Check sheet for the drawn part. Datum: minimum x, y, z corner. Units: mm. A direction names the side the tool comes from. Coordinates: 2 decimals unless noted, no trailing zeros. Loops run counter-clockwise (first coordinate to the right, second up) from the corner with the lowest first, then second, coordinate; pieces in that order, holes last.
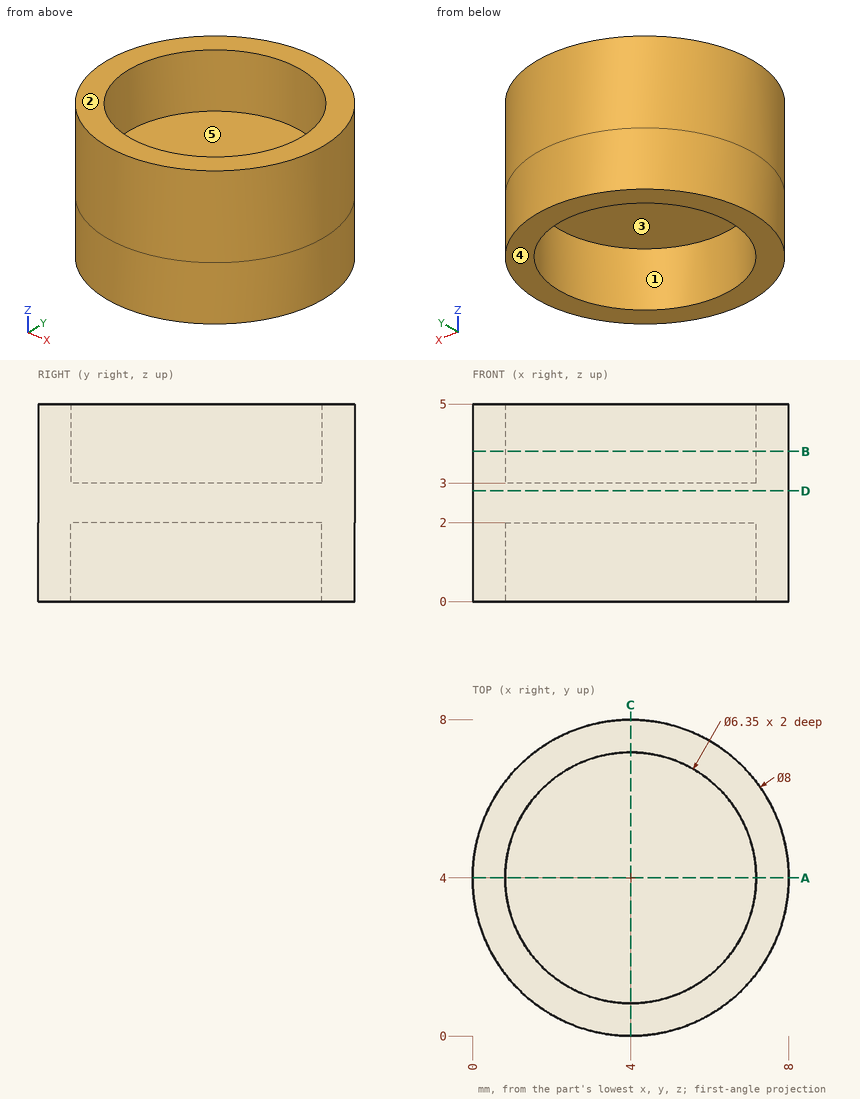
1) Section check A-A on y = 4. Enter the section's corners in (x, z) (3 decimals), plus the area to 3 significant figures.
Answer sheet:
outline: (0, 0) - (0.825, 0) - (0.825, 2) - (7.175, 2) - (7.175, 0) - (8, 0) - (8, 5) - (7.175, 5) - (7.175, 3) - (0.825, 3) - (0.825, 5) - (0, 5) - close
area: 14.6 mm2
2) Section check D-D on z = 2.8. Enter the section's corners in (x, y).
Answer sheet:
outline: circle Ø8 at (4, 4)
3) Depth check by flat-ended pin: pin 1 (1.9 mm diameter, centred on x = 5.5, y = 3, fed in from +Z); pin 2 (1 mm diameter, centred on x = 4.5, y = 5, fed in from -Z); pin 3 (2 mm diameter, centred on x = 7, z = 3, fed in from -Y). Enter the tip coordinate at first touch or a pass-through.
Answer sheet:
pin 1: stops at z = 3
pin 2: stops at z = 2
pin 3: stops at y = 0.54
4) Mould release check, pull along X, two halves, no side actions. Record for the marked faces 1, 2 and 3: +X half, -X half, draft (parallel to the pull), parting line (faces both ways), or undercut.
Answer sheet:
face 1: undercut
face 2: draft
face 3: undercut
5) Set-up check for the marked faces 4 and 5: record each of +Z, -Z, +X, -X, +Y, -Y from which the full face is reachable in a straight line by a thin tool's end or side.
Answer sheet:
face 4: -Z, +X, -X, +Y, -Y
face 5: +Z
6) Scan lines: line 1 (Y direction, x = 4, z = 3.5) (3 decimals); line 2 (Y direction, x = 6.5, z = 3.65); line 3 (X direction, y = 6.75, z = 3.05). Record each from-to range of solid material in increasing order.
Answer sheet:
line 1: y = 0 to 0.825, 7.175 to 8
line 2: y = 0.88 to 2.04, 5.96 to 7.12
line 3: x = 1.1 to 2.41, 5.59 to 6.9
7) Section check B-B on z = 3.8. Enter the section's corners in (x, y) (3 decimals).
Answer sheet:
outline: circle Ø8 at (4, 4); hole circle Ø6.35 at (4, 4)
